Design review of the part built by this model. Coordinates are the model's own, in mm. Give positions to 0.01 mm unless a question says otherwise; leave off trailing zeros.
```python
from build123d import *

# Parameters (mm, degrees)
F0_R     = 76.2
F1_DEPTH = 52.07
F2_R     = 5.08
F3_R     = 5.3715880148
F3_R_2   = 4.2370614404
F3_R_3   = 6.3108884309
F3_R_4   = 3.8766310323
F3_R_5   = 4.6528327754
F3_R_6   = 3.1865727254
F3_R_7   = 5.0301198982
F3_R_8   = 4.907734168
F3_R_9   = 9.4320215761
F3_R_10  = 8.4400514289
F3_R_11  = 5.3159973794
F3_R_12  = 4.9419144622
F3_R_13  = 5.7632073099
F3_R_14  = 10.3738042339
F3_R_15  = 5.05451088
F3_R_16  = 3.0558865435
F4_DEPTH = 52.0710001


with BuildPart() as f1:
    # F0 (on Top) → F1 (new body)
    with BuildSketch(Plane.XY):
        Circle(F0_R)
    extrude(amount=F1_DEPTH)

    # F2
    f2_edges = [f1.edges().sort_by_distance(p)[0] for p in [
        (-76.2, 0, 0),
        (-76.2, 0, 52.07),
    ]]
    fillet(f2_edges, radius=F2_R)

    # F3 (on face) → F4 (cut, through all)
    with BuildSketch(Plane.XY.offset(52.07)):
        with BuildLine():
            ThreePointArc((-37.009803901, -23.6505497776), (-41.4263644142, -21.2516242438), (-44.7620251929, -17.4920740509))
            ThreePointArc((-44.7620251929, -17.4920740509), (-48.0466092381, -17.1106960922), (-51.3124818641, -17.6284001476))
            ThreePointArc((-51.3124818641, -17.6284001476), (-52.8076132814, -19.5680988122), (-55.2546881101, -19.6664535121))
            ThreePointArc((-55.2546881101, -19.6664535121), (-53.1375621362, -40.1879116404), (-35.6350277314, -29.2666591704))
            ThreePointArc((-35.6350277314, -29.2666591704), (-35.9837218408, -26.375695048), (-37.009803901, -23.6505497776))
        make_face()
        with Locations((-22.6189903915, 19.9577584863)):
            Circle(F3_R)
        with Locations((-38.4934768081, 46.9580106437)):
            Circle(F3_R_2)
        with Locations((-43.1242734194, 26.2293871492)):
            Circle(F3_R_3)
        with Locations((-8.4645338356, 40.1057675481)):
            Circle(F3_R_4)
        with Locations((9.4722164795, 47.361087054)):
            Circle(F3_R_5)
        with Locations((-3.0230483972, 61.468642205)):
            Circle(F3_R_6)
        with Locations((10.4064103216, 17.884016037)):
            Circle(F3_R_7)
        with Locations((37.2842587531, 26.8043577671)):
            Circle(F3_R_8)
        with Locations((18.2558577508, -9.1234976426)):
            Circle(F3_R_9)
        with Locations((37.6561321318, -16.9201008976)):
            Circle(F3_R_10)
        with Locations((33.640883863, -41.6150391102)):
            Circle(F3_R_11)
        with Locations((18.300132826, -41.7637899518)):
            Circle(F3_R_12)
        with Locations((-5.0592576154, -30.087729916)):
            Circle(F3_R_13)
        with Locations((-29.7136716545, -43.0898442864)):
            Circle(F3_R_14)
        with Locations((34.0596735477, 40.1057675481)):
            Circle(F3_R_15)
        with Locations((-59.3534111977, 4.7666169703)):
            Circle(F3_R_16)
    extrude(amount=-F4_DEPTH, mode=Mode.SUBTRACT)


solid = f1.part
```
1. Take a section at A-A (z = 29). State how many separate pieces and enclosed holes the cut face has, then the cut area to 3 significant figures.
Recorded:
separate pieces: 1
enclosed holes: 17
area: 16,000 mm2
2. For line 1 along Y through (x, z) = (8, 41); line 2 along X through (y, z) = (31, 33); line 3 along X through (y, z) = (-44, 29.5), list the stretches that pass through material, from the lowest coordinate up.
Recorded:
line 1: y = -75.78 to 13.47, 22.3 to 42.95, 51.77 to 75.78
line 2: x = -69.61 to -47.26, -38.99 to 34.74, 39.83 to 69.61
line 3: x = -62.21 to -40.05, -19.38 to 13.89, 22.71 to 28.89, 38.39 to 62.21
3. For pin 1 (7.5 mm diameter, centred on x = 9.47, y = 47.36, fed in from +Z); pin 2 (8 mm diameter, centred on y = 60, z = 29.5, fed in from -X); pin 3 (4 mm diameter, centred on x = -46.5, z = 36, fed in from -Y); pin 4 (15.5 mm diameter, centred on x = 37.28, y = 26.8, fed in from +Z), all flat-tipped, find the tip position at first contact; note any pin that passes through.
Recorded:
pin 1: passes through
pin 2: stops at x = -51.68
pin 3: stops at y = -61.86
pin 4: stops at z = 52.07
4. Draft analysis for pull direction Y (two halves, no side actions). For faces 1 (the face through (-1, 1, 52.07)), 2 (the face through (-60.47, -46.367, 25.742)), 3 (the face through (12.728, 13.421, 26.399)), state which applies: pulls with the +Y half, pulls with the -Y half, needs draft (parallel to the pull), parting line crosses it, or undercut.
Recorded:
face 1: needs draft
face 2: parting line crosses it
face 3: undercut
